from build123d import *

# Parameters (mm, degrees)
SKETCH1_W           = 414
SKETCH1_H           = 164
BOSS_EXTRUDE1_DEPTH = 3
SKETCH2_W           = 3
SKETCH2_H           = 11
SKETCH2_H_2         = 12
CUT_EXTRUDE1_DEPTH  = 3
CUT_EXTRUDE2_DEPTH  = 3
SKETCH4_R           = 1.5
SKETCH4_W           = 3
SKETCH4_H           = 10
CUT_EXTRUDE3_DEPTH  = 10
CUT_EXTRUDE4_DEPTH  = 10


with BuildPart() as part:
    # Sketch1 → Boss-Extrude1 (new body)
    with BuildSketch(Plane.XY.offset(152)):
        Rectangle(SKETCH1_W, SKETCH1_H)
    extrude(amount=BOSS_EXTRUDE1_DEPTH)

    # Sketch2 → Cut-Extrude1 (cut)
    with BuildSketch(Plane.ZY.offset(207)):
        with Locations((153.5, -76.5)):
            Rectangle(SKETCH2_W, SKETCH2_H)
        with Locations((153.5, -55)):
            Rectangle(SKETCH2_W, SKETCH2_H_2)
        with Locations((153.5, -33)):
            Rectangle(SKETCH2_W, SKETCH2_H_2)
        with Locations((153.5, -11)):
            Rectangle(SKETCH2_W, SKETCH2_H_2)
        with Locations((153.5, 11)):
            Rectangle(SKETCH2_W, SKETCH2_H_2)
        with Locations((153.5, 33)):
            Rectangle(SKETCH2_W, SKETCH2_H_2)
        with Locations((153.5, 55)):
            Rectangle(SKETCH2_W, SKETCH2_H_2)
        with Locations((153.5, 76.5)):
            Rectangle(SKETCH2_W, SKETCH2_H)
    cut_extrude1 = extrude(amount=-CUT_EXTRUDE1_DEPTH, mode=Mode.SUBTRACT)

    # Mirror1: Cut-Extrude1 across plane
    add(cut_extrude1.mirror(Plane(origin=(0, 0, 0), x_dir=(0, 0, 1), z_dir=(1, 0, 0))), mode=Mode.SUBTRACT)

    # Sketch3 → Cut-Extrude2 (cut)
    with BuildSketch(Plane(origin=(0, 82, 0), x_dir=(1, 0, 0), z_dir=(0, 1, 0))):
        Polygon((174, -152), (194, -152), (194, -155), (204, -155), (204, -145), (207, -145), (207, -133), (204, -133), (204, -123), (207, -123), (207, -111), (204, -111), (204, -101), (207, -101), (207, -89), (204, -89), (204, -79), (207, -79), (207, -67), (204, -67), (204, -57), (207, -57), (207, -45), (204, -45), (204, -35), (207, -35), (207, -23), (204, -23), (204, -16), (-204, -16), (-204, -23), (-207, -23), (-207, -35), (-204, -35), (-204, -45), (-207, -45), (-207, -57), (-204, -57), (-204, -67), (-207, -67), (-207, -79), (-204, -79), (-204, -89), (-207, -89), (-207, -101), (-204, -101), (-204, -111), (-207, -111), (-207, -123), (-204, -123), (-204, -133), (-207, -133), (-207, -145), (-204, -145), (-204, -155), (-186, -155), (-186, -152), (-166, -152), (-166, -155), (-146, -155), (-146, -152), (-126, -152), (-126, -155), (-106, -155), (-106, -152), (-86, -152), (-86, -155), (-66, -155), (-66, -152), (-46, -152), (-46, -155), (-26, -155), (-26, -152), (-6, -152), (-6, -155), (14, -155), (14, -152), (34, -152), (34, -155), (54, -155), (54, -152), (74, -152), (74, -155), (94, -155), (94, -152), (114, -152), (114, -155), (134, -155), (134, -152), (154, -152), (154, -155), (174, -155), align=None)
    cut_extrude2 = extrude(amount=-CUT_EXTRUDE2_DEPTH, mode=Mode.SUBTRACT)

    # Mirror2: Cut-Extrude2 across plane
    add(cut_extrude2.mirror(Plane.ZX), mode=Mode.SUBTRACT)

    # Sketch4 → Cut-Extrude3 (cut)
    with BuildSketch(Plane.XY.offset(155)):
        with Locations((139, 37)):
            Circle(SKETCH4_R)
        with Locations((195, 37)):
            Circle(SKETCH4_R)
        with Locations((195, 77)):
            Circle(SKETCH4_R)
        with Locations((139, 77)):
            Circle(SKETCH4_R)
        with Locations((-78, 77)):
            Circle(SKETCH4_R)
        with Locations((-22, 77)):
            Circle(SKETCH4_R)
        with Locations((-78, 37)):
            Circle(SKETCH4_R)
        with Locations((-22, 37)):
            Circle(SKETCH4_R)
        with Locations((139, -77)):
            Circle(SKETCH4_R)
        with Locations((195, -77)):
            Circle(SKETCH4_R)
        with Locations((195, -37)):
            Circle(SKETCH4_R)
        with Locations((139, -37)):
            Circle(SKETCH4_R)
        with Locations((-22, -37)):
            Circle(SKETCH4_R)
        with Locations((-78, -37)):
            Circle(SKETCH4_R)
        with Locations((-22, -77)):
            Circle(SKETCH4_R)
        with Locations((-78, -77)):
            Circle(SKETCH4_R)
        with Locations((-133.5, 22)):
            Rectangle(SKETCH4_W, SKETCH4_H)
        with Locations((-133.5, 0)):
            Rectangle(SKETCH4_W, SKETCH4_H)
        with Locations((-133.5, -22)):
            Rectangle(SKETCH4_W, SKETCH4_H)
        with Locations((108.5, 22)):
            Rectangle(SKETCH4_W, SKETCH4_H)
        with Locations((108.5, 0)):
            Rectangle(SKETCH4_W, SKETCH4_H)
        with Locations((108.5, -22)):
            Rectangle(SKETCH4_W, SKETCH4_H)
    extrude(amount=-CUT_EXTRUDE3_DEPTH, mode=Mode.SUBTRACT)

    # Sketch5 → Cut-Extrude4 (cut)
    with BuildSketch(Plane.XY.offset(155)):
        with BuildLine():
            Line((-34.7, 4.6), (-18.7, 4.6))
            ThreePointArc((-18.7, 4.6), (-13.750252532, 6.650252532), (-11.7, 11.6))
            Line((-11.7, 11.6), (-11.7, 12.6))
            ThreePointArc((-11.7, 12.6), (-13.750252532, 17.549747468), (-18.7, 19.6))
            Line((-18.7, 19.6), (-34.7, 19.6))
            ThreePointArc((-34.7, 19.6), (-39.649747468, 17.549747468), (-41.7, 12.6))
            Line((-41.7, 12.6), (-41.7, 11.6))
            ThreePointArc((-41.7, 11.6), (-39.649747468, 6.650252532), (-34.7, 4.6))
        make_face()
    extrude(amount=-CUT_EXTRUDE4_DEPTH, mode=Mode.SUBTRACT)


solid = part.part
Geometry check sheet. Reference: the model listing, model coordinates, mm. A direction names the side the tool comes from. Give positions to 0.01 mm unless a question says otherwise; leave off trailing zeros. Answer as a JSON object with one key per item and string values. Group by question number.
Item 1: Sectioned sample at A-A on z = 152.5. Give the number of separate pieces and of enclosed holes in the cut face, plus the area to 3 significant figures.
Item 2: Material ranges on L1, parallel to X at y = 22, z = 154.5; L2, parallel to X at y = -77, z = 153.7; L3, parallel to Y at x = 195, z = 153.8, recorded low to high.
Item 3: Access from +Z, -Z, +X, -X, +Y, -Y to the whole of each face (thin tool, end or side, straight path). Record for faces 1 (the cylindrical face through (-13.8, 6.6, 153.5)), 2 (the flat face through (-3, 1, 152)).
Item 4: Gauge pin test, flat ends, axial feed: pin 1 (0.9 mm diameter, centred on y = -32.5, z = 153, fed in from +X); pin 2 (1.5 mm diameter, centred on y = 60, z = 154, fed in from -X); pin 3 (0.9 mm diameter, centred on x = 82, z = 153, fed in from +Y). Record the tip position at first contact, or that the pin passes through.
Item 5: Mould release check, pull along X, two halves, no side actions. Record for faces 3 (the cylindrical face through (-39.7, 6.7, 153.5)), 4 (the flat face through (-3, 1, 155)), 5 (the cylindrical face through (-13.7, 17.5, 153.5)): pulls with the +X half, pulls with the -X half, needs draft (parallel to the pull), parting line crosses it, or undercut.
Findings below:
{
 "1": {"separate pieces": "1", "enclosed holes": "23", "area": "65,400 mm2"},
 "2": {"L1": "-207 to -135, -132 to 107, 110 to 207", "L2": "-204 to -79.5, -76.5 to -23.5, -20.5 to 137.5, 140.5 to 193.5, 196.5 to 204", "L3": "-79 to -78.5, -75.5 to -38.5, -35.5 to 35.5, 38.5 to 75.5, 78.5 to 79"},
 "3": {"face 1": "+Z, -Z", "face 2": "-Z, +X, -X, +Y, -Y"},
 "4": {"pin 1": "x = 204", "pin 2": "x = -204", "pin 3": "y = 79"},
 "5": {"face 3": "undercut", "face 4": "needs draft", "face 5": "undercut"}
}
